Read the model definition and answer for the solid it produces. Units are mm, in the model's axes. Coordinates: 2 decimals unless noted, no trailing zeros. Order: outer loops, then holes, each group sorted by start corner. A loop starts at its lowest first (then second) coordinate and runs counter-clockwise, first axis right, second up.
```python
from build123d import *

# Parameters (mm, degrees)
F0_R     = 11.15
F1_DEPTH = 10


with BuildPart() as f1:
    # F0 (on Top) → F1 (new body)
    with BuildSketch(Plane.XY):
        with BuildLine():
            ThreePointArc((38.44596875, -11.0411723505), (28.85, 0), (38.44596875, 11.0411723505))
            ThreePointArc((38.44596875, 11.0411723505), (35.883662554, 17.6737874184), (32.1875, 23.74794399))
            ThreePointArc((32.1875, 23.74794399), (15, 0), (32.1875, -23.74794399))
            ThreePointArc((32.1875, -23.74794399), (35.883662554, -17.6737874184), (38.44596875, -11.0411723505))
        make_face()
        with BuildLine():
            ThreePointArc((32.1875, 23.74794399), (35.883662554, 17.6737874184), (38.44596875, 11.0411723505))
            ThreePointArc((38.44596875, 11.0411723505), (47.3142002831, 8.4157574952), (51.15, 0))
            ThreePointArc((51.15, 0), (47.3142002831, -8.4157574952), (38.44596875, -11.0411723505))
            ThreePointArc((38.44596875, -11.0411723505), (35.883662554, -17.6737874184), (32.1875, -23.74794399))
            ThreePointArc((32.1875, -23.74794399), (54.6575492494, -20.2523146825), (65, 0))
            ThreePointArc((65, 0), (54.6575492494, 20.2523146825), (32.1875, 23.74794399))
        make_face()
        with BuildLine():
            ThreePointArc((32.1875, -23.74794399), (15, 0), (32.1875, 23.74794399))
            ThreePointArc((32.1875, 23.74794399), (28.2842712475, 28.2842712475), (23.74794399, 32.1875))
            ThreePointArc((23.74794399, 32.1875), (0, 15), (-23.74794399, 32.1875))
            ThreePointArc((-23.74794399, 32.1875), (-28.2842712475, 28.2842712475), (-32.1875, 23.74794399))
            ThreePointArc((-32.1875, 23.74794399), (-19.7476853175, 14.6575492494), (-15, 0))
            ThreePointArc((-15, 0), (-19.7476853175, -14.6575492494), (-32.1875, -23.74794399))
            ThreePointArc((-32.1875, -23.74794399), (-28.2842712475, -28.2842712475), (-23.74794399, -32.1875))
            ThreePointArc((-23.74794399, -32.1875), (0, -15), (23.74794399, -32.1875))
            ThreePointArc((23.74794399, -32.1875), (28.2842712475, -28.2842712475), (32.1875, -23.74794399))
        make_face()
        Circle(F0_R, mode=Mode.SUBTRACT)
        with BuildLine():
            ThreePointArc((-23.74794399, 32.1875), (0, 15), (23.74794399, 32.1875))
            ThreePointArc((23.74794399, 32.1875), (17.6737874184, 35.883662554), (11.0411723505, 38.44596875))
            ThreePointArc((11.0411723505, 38.44596875), (0, 28.85), (-11.0411723505, 38.44596875))
            ThreePointArc((-11.0411723505, 38.44596875), (-17.6737874184, 35.883662554), (-23.74794399, 32.1875))
        make_face()
        with BuildLine():
            ThreePointArc((11.0411723505, 38.44596875), (17.6737874184, 35.883662554), (23.74794399, 32.1875))
            ThreePointArc((23.74794399, 32.1875), (24.6850015166, 36.0439034231), (25, 40))
            ThreePointArc((25, 40), (-3.9560965769, 64.6850015166), (-23.74794399, 32.1875))
            ThreePointArc((-23.74794399, 32.1875), (-17.6737874184, 35.883662554), (-11.0411723505, 38.44596875))
            ThreePointArc((-11.0411723505, 38.44596875), (-0.7789185746, 51.1227598128), (11.15, 40))
            ThreePointArc((11.15, 40), (11.1227598128, 39.2210814254), (11.0411723505, 38.44596875))
        make_face()
        with BuildLine():
            ThreePointArc((25, -40), (24.6850015166, -36.0439034231), (23.74794399, -32.1875))
            ThreePointArc((23.74794399, -32.1875), (17.6737874184, -35.883662554), (11.0411723505, -38.44596875))
            ThreePointArc((11.0411723505, -38.44596875), (11.1227598128, -39.2210814254), (11.15, -40))
            ThreePointArc((11.15, -40), (-0.7789185746, -51.1227598128), (-11.0411723505, -38.44596875))
            ThreePointArc((-11.0411723505, -38.44596875), (-17.6737874184, -35.883662554), (-23.74794399, -32.1875))
            ThreePointArc((-23.74794399, -32.1875), (-3.9560965769, -64.6850015166), (25, -40))
        make_face()
        with BuildLine():
            ThreePointArc((11.0411723505, -38.44596875), (17.6737874184, -35.883662554), (23.74794399, -32.1875))
            ThreePointArc((23.74794399, -32.1875), (0, -15), (-23.74794399, -32.1875))
            ThreePointArc((-23.74794399, -32.1875), (-17.6737874184, -35.883662554), (-11.0411723505, -38.44596875))
            ThreePointArc((-11.0411723505, -38.44596875), (0, -28.85), (11.0411723505, -38.44596875))
        make_face()
        with BuildLine():
            ThreePointArc((-15, 0), (-19.7476853175, 14.6575492494), (-32.1875, 23.74794399))
            ThreePointArc((-32.1875, 23.74794399), (-35.883662554, 17.6737874184), (-38.44596875, 11.0411723505))
            ThreePointArc((-38.44596875, 11.0411723505), (-31.5842425048, 7.3142002831), (-28.85, 0))
            ThreePointArc((-28.85, 0), (-31.5842425048, -7.3142002831), (-38.44596875, -11.0411723505))
            ThreePointArc((-38.44596875, -11.0411723505), (-35.883662554, -17.6737874184), (-32.1875, -23.74794399))
            ThreePointArc((-32.1875, -23.74794399), (-19.7476853175, -14.6575492494), (-15, 0))
        make_face()
        with BuildLine():
            ThreePointArc((-38.44596875, 11.0411723505), (-35.883662554, 17.6737874184), (-32.1875, 23.74794399))
            ThreePointArc((-32.1875, 23.74794399), (-65, 0), (-32.1875, -23.74794399))
            ThreePointArc((-32.1875, -23.74794399), (-35.883662554, -17.6737874184), (-38.44596875, -11.0411723505))
            ThreePointArc((-38.44596875, -11.0411723505), (-51.15, 0), (-38.44596875, 11.0411723505))
        make_face()
    extrude(amount=F1_DEPTH)


solid = f1.part
```
1) A cutting plane is placed at C-C, the plane y = 47. Determine the outline of the cut face in (x, z), and give its area (3 significant figures).
A:
outline: (-24, 0) - (-8.68, 0) - (-8.68, 10) - (-24, 10) - close; (8.68, 0) - (24, 0) - (24, 10) - (8.68, 10) - close
area: 306 mm2
2) A cutting plane is placed at A-A, the plane x = 40. Determine the outline of the cut face in (y, z), and give its area (3 significant figures).
A:
outline: (-25, 0) - (-11.15, 0) - (-11.15, 10) - (-25, 10) - close; (11.15, 0) - (25, 0) - (25, 10) - (11.15, 10) - close
area: 277 mm2
3) A cutting plane is placed at B-B, the plane z = 5. Determine the outline of the cut face in (x, y), and give its area (3 significant figures).
A:
outline: (-32.19, -23.75) arc R40 ccw to (-23.75, -32.19) arc R25 ccw (long way) to (23.75, -32.19) arc R40 ccw to (32.19, -23.75) arc R25 ccw (long way) to (32.19, 23.75) arc R40 ccw to (23.75, 32.19) arc R25 ccw (long way) to (-23.75, 32.19) arc R40 ccw to (-32.19, 23.75) arc R25 ccw (long way) to start; hole circle Ø22.3 at (-40, 0); hole circle Ø22.3 at (0, -40); hole circle Ø22.3 at (0, 0); hole circle Ø22.3 at (0, 40); hole circle Ø22.3 at (40, 0)
area: 7,530 mm2
4) Straight lines are drawn through the part: line 1 (Y direction, x = 0, z = 7); line 2 (Y direction, x = 40, z = 7). For each, find the intervals that lie inside material, in ascending order.
A:
line 1: y = -65 to -51.15, -28.85 to -11.15, 11.15 to 28.85, 51.15 to 65
line 2: y = -25 to -11.15, 11.15 to 25
5) Determine the mould class of faces 1 (the cylindrical face through (10.635, 3.349, 4.93)), 2 (the flat face through (14, 1, 10)) for opening direction X: pulls with the +X half, pulls with the -X half, needs draft (parallel to the pull), parting line crosses it, or undercut.
A:
face 1: undercut
face 2: needs draft
6) Flat-ended cylindrical pins translate along their axes: pin 1 Ø18 at (x, y) = (-40, 0) entering from -Z; pin 2 Ø6 at (x, z) = (-36.5, 7.5) entering from +Y (3 decimals); pin 3 Ø3 at (x, z) = (-39.5, 9) entering from -Y; pin 4 Ø6 at (y, z) = (-38, 2) entering from -X. Find the tip coordinate at first contact, or state that the pin passes through.
A:
pin 1: passes through
pin 2: stops at y = 24.995
pin 3: stops at y = -25
pin 4: stops at x = -25
7) A cutting plane is placed at D-D, the plane x = 0. Determine the outline of the cut face in (y, z), and give its area (3 significant figures).
A:
outline: (-65, 0) - (-51.15, 0) - (-51.15, 10) - (-65, 10) - close; (-28.85, 0) - (-11.15, 0) - (-11.15, 10) - (-28.85, 10) - close; (11.15, 0) - (28.85, 0) - (28.85, 10) - (11.15, 10) - close; (51.15, 0) - (65, 0) - (65, 10) - (51.15, 10) - close
area: 631 mm2
